Drawing for the job (mm, zero at the part's lowest x, y, z). Give positions to 0.01 mm unless a question says otherwise; leave off trailing zeros. Order: outer loops, then holes, each group sorted by start corner. A loop starts at its lowest first (then second) coordinate and runs counter-clockwise, first axis right, second up. Notation, with made-up numbers: (5.25, 28) -> (51.25, 28) arc R16 cw to (51.25, 59) -> close; hole circle Ø3 at (63, 8). An arc over 180 degrees is marked (long way). One line per item, written item: value. Start each with the question number.
(1) Saw through at B-B on y = 0.35. Give the cut face in (x, z), plus the area to 3 significant figures.
(2) Saw through at A-A on x = 6.35. Give the cut face in (y, z).
(3) Saw through at C-C on x = 95.25. Give the cut face in (y, z).
(4) Probe line 1 (X direction, y = 0.95, z = 6.25); line 2 (Z direction, x = 95.25, y = 1.2); line 3 (Z direction, x = 177.8, y = 1.3) (1 decimal). List the from-to ranges inside material, lowest first.
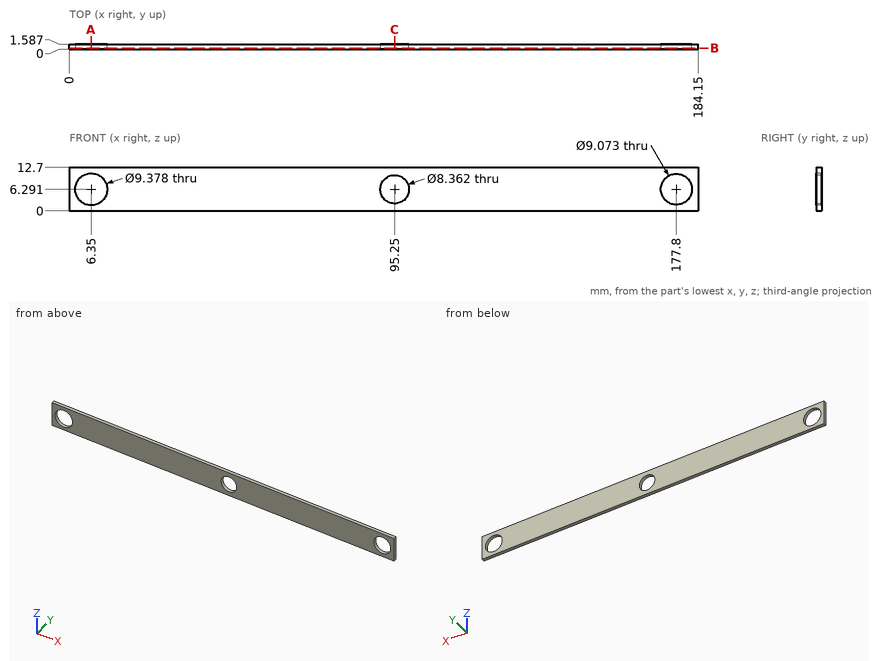
Results below:
1. outline: (0, 0) -> (184.15, 0) -> (184.15, 12.7) -> (0, 12.7) -> close; hole circle Ø9.38 at (6.35, 6.29); hole circle Ø8.36 at (95.25, 6.29); hole circle Ø9.07 at (177.8, 6.29)
1. area: 2,150 mm²
2. outline: (0, 0) -> (1.59, 0) -> (1.59, 1.6) -> (0, 1.6) -> close; (0, 10.98) -> (1.59, 10.98) -> (1.59, 12.7) -> (0, 12.7) -> close
3. outline: (0, 0) -> (1.59, 0) -> (1.59, 2.11) -> (0, 2.11) -> close; (0, 10.47) -> (1.59, 10.47) -> (1.59, 12.7) -> (0, 12.7) -> close
4. line 1: x = 0 to 1.66, 11.04 to 91.07, 99.43 to 173.26, 182.34 to 184.15
4. line 2: z = 0 to 2.11, 10.47 to 12.7
4. line 3: z = 0 to 1.8, 10.8 to 12.7
